The model under review builds one solid part; all positions refer to its coordinate system, in mm. A direction names the side the tool comes from. Give positions to 0.01 mm unless a question says otherwise; leave off trailing zeros. Loops run counter-clockwise (first coordinate to the right, second up) from the corner with the lowest first, then second, coordinate; pieces in that order, holes last. Notation, with made-up numbers: M 59.25,66.25 L 100.25,66.25 A18 ccw 100.25,92.25 Z; hole C 30,52.25 d5. An arc over 180 degrees is marked long. Return JSON: item names as keys, results as strings.
```python
from build123d import *

# Parameters (mm, degrees)
BOSS_EXTRUDE1_DEPTH      = 8
SKETCH2_R                = 1.5
CUT_EXTRUDE1_DEPTH       = 10
SKETCH3_R                = 1.5
CUT_EXTRUDE2_DEPTH       = 10
BOSS_EXTRUDE3_DEPTH      = 30
BOSS_EXTRUDE3_DEPTH_BACK = 8
SKETCH6_W                = 20
SKETCH6_H                = 10
FILLET3_R                = 12
SKETCH7_W                = 20
SKETCH7_H                = 30
BOSS_EXTRUDE4_DEPTH      = 2
CUT_EXTRUDE3_DEPTH       = 10
SKETCH9_R                = 5.5
CUT_EXTRUDE4_DEPTH       = 10
FILLET4_R                = 5
FILLET5_R                = 2


with BuildPart() as part:
    # Sketch1 → Boss-Extrude1 (new body)
    with BuildSketch(Plane.XY):
        with BuildLine():
            Line((-25, 10), (40, 10))
            ThreePointArc((40, 10), (50, 0), (40, -10))
            Line((40, -10), (-25, -10))
            Line((-25, -10), (-25, 10))
        make_face()
    extrude(amount=BOSS_EXTRUDE1_DEPTH)

    # Sketch2 → Cut-Extrude1 (cut)
    with BuildSketch(Plane.XY.offset(8)):
        with Locations((40, 0)):
            Circle(SKETCH2_R)
    extrude(amount=-CUT_EXTRUDE1_DEPTH, mode=Mode.SUBTRACT)

    # Sketch3 → Cut-Extrude2 (cut)
    with BuildSketch(Plane(origin=(0, 0, 0), x_dir=(-1, 0, 0), z_dir=(0, 0, -1))):
        with Locations((-15, 0)):
            Circle(SKETCH3_R)
    extrude(amount=-CUT_EXTRUDE2_DEPTH, mode=Mode.SUBTRACT)

    # Sketch6 → Boss-Extrude3 (add, two sides: drawn at the far end of the back side and taken through both)
    with BuildSketch(Plane(origin=(0, 0, 0), x_dir=(-1, 0, 0), z_dir=(0, 0, -1)).offset(-BOSS_EXTRUDE3_DEPTH_BACK)):
        with Locations((15, -15)):
            Rectangle(SKETCH6_W, SKETCH6_H)
    extrude(amount=BOSS_EXTRUDE3_DEPTH + BOSS_EXTRUDE3_DEPTH_BACK)

    # Fillet3
    # the kernel refuses this fillet: 12 mm, written as the material it adds along each edge
    with BuildSketch(Plane(origin=(-5, -10, 8), x_dir=(0, -1, 0), z_dir=(0, 0, -1))) as fillet3_piece_1:
        with BuildLine():
            CenterArc((12, -11.832159566), FILLET3_R, 99.594068227, 80.405931773)
            Line((0, -11.832159566), (0, 0))
            Line((0, 0), (10, 0))
        make_face()
    extrude(amount=8)

    # Sketch7 → Boss-Extrude4 (add)
    with BuildSketch(Plane(origin=(0, -10, 0), x_dir=(1, 0, 0), z_dir=(0, 1, 0))):
        with Locations((-15, 15)):
            Rectangle(SKETCH7_W, SKETCH7_H)
    extrude(amount=BOSS_EXTRUDE4_DEPTH)

    # Sketch8 → Cut-Extrude3 (cut)
    with BuildSketch(Plane.XZ.offset(20)):
        Polygon((-12.092828782, -7.012612723), (-20.463694682, -8.488622233), (-23.370865901, -16.47600951), (-17.907171218, -22.987387277), (-9.536305318, -21.511377767), (-6.629134099, -13.52399049), align=None)
    extrude(amount=-CUT_EXTRUDE3_DEPTH, mode=Mode.SUBTRACT)

    # Sketch9 → Cut-Extrude4 (cut)
    with BuildSketch(Plane.XZ.offset(10)):
        with Locations(Location((-15, -15, 0), (0, 0, 270))):
            Circle(SKETCH9_R)
    extrude(amount=-CUT_EXTRUDE4_DEPTH, mode=Mode.SUBTRACT)

    # Fillet4
    # the kernel refuses this fillet: 5 mm, written as the material it adds along each edge
    with BuildSketch(Plane(origin=(-5, -20, 0), x_dir=(1, 0, 0), z_dir=(0, 1, 0))) as fillet4_piece_1_section:
        with BuildLine():
            CenterArc((FILLET4_R, FILLET4_R), FILLET4_R, 180, 90)
            Line((0, FILLET4_R), (0, 0))
            Line((0, 0), (FILLET4_R, 0))
        make_face()
    fillet4_piece_1 = extrude(amount=12, mode=Mode.PRIVATE)
    fillet4_piece_1 = fillet4_piece_1 - Plane(origin=(6.832159566, -22, 0), x_dir=(0, -1, 0), z_dir=(0, 0, 1)) * Cylinder(12, 44, mode=Mode.PRIVATE)
    add(fillet4_piece_1)
    with BuildSketch(Plane(origin=(-25, -8, 0), x_dir=(0, 1, 0), z_dir=(1, 0, 0))) as fillet4_piece_2:
        with BuildLine():
            CenterArc((FILLET4_R, -FILLET4_R), FILLET4_R, 90, 90)
            Line((0, -FILLET4_R), (0, 0))
            Line((0, 0), (FILLET4_R, 0))
        make_face()
    extrude(amount=20)
    with BuildSketch(Plane(origin=(-5, -20, 0), x_dir=(1, 0, 0), z_dir=(0, 1, 0))) as fillet4_piece_3a_section:
        with BuildLine():
            CenterArc((FILLET4_R, FILLET4_R), FILLET4_R, 180, 90)
            Line((0, FILLET4_R), (0, 0))
            Line((0, 0), (FILLET4_R, 0))
        make_face()
    fillet4_piece_3a = extrude(amount=24.5, mode=Mode.PRIVATE)
    fillet4_piece_3a = split(fillet4_piece_3a, bisect_by=Plane(origin=(-5, -8, 0), z_dir=(0, 1, 0)), keep=Keep.TOP, mode=Mode.PRIVATE)
    with BuildSketch(Plane(origin=(-25, -8, 0), x_dir=(0, 1, 0), z_dir=(1, 0, 0))) as fillet4_piece_3b_section:
        with BuildLine():
            CenterArc((FILLET4_R, -FILLET4_R), FILLET4_R, 90, 90)
            Line((0, -FILLET4_R), (0, 0))
            Line((0, 0), (FILLET4_R, 0))
        make_face()
    fillet4_piece_3b = extrude(amount=32.5, mode=Mode.PRIVATE)
    fillet4_piece_3b = split(fillet4_piece_3b, bisect_by=Plane(origin=(-5, -8, 0), z_dir=(1, 0, 0)), keep=Keep.TOP, mode=Mode.PRIVATE)
    fillet4_piece_3 = fillet4_piece_3a & fillet4_piece_3b
    add(fillet4_piece_3)

    # Fillet5
    fillet5_edges = [part.edges().sort_by_distance(p)[0] for p in [
        (-15, -20, 8),
        (-25, -14, -30),
        (-5, -14, -30),
        (-25, 10, 4),
    ]]
    fillet(fillet5_edges, radius=FILLET5_R)


solid = part.part
```
1) Consider section B-B on z = -15. Write out the cut boundary in (x, y).
From the geometry:
{"outline": "M -25,-20 L -22.83,-20 L -22.83,-10 L -20.5,-10 L -20.5,-8 L -25,-8 Z; M -9.5,-10 L -7.17,-10 L -7.17,-20 L -5,-20 L -5,-8 L -9.5,-8 Z"}
2) Wall thickness on L1, parallel to Y at x = 15, z = 2; L2, parallel to X at y = -8.9, z = -15; L3, parallel to Y at x = 8, z = 3.5: over which ranges is each line inside the solid? List them lowest first. Write a range as from..to.
From the geometry:
{"L1": "-10..-1.5, 1.5..10", "L2": "-25..-20.5, -9.5..-5", "L3": "-10..10"}
3) The part is to be moulded in two halves that separate along Z. For faces 4 (the face through (-24.43, -14.08, -29.4)), 5 (the face through (-8.1, -15.07, -17.57)), 6 (the face through (-25, -12, -6)), say which applies: released by +Z, released by -Z, zero draft, split by the parting line, or undercut.
From the geometry:
{"face 4": "released by -Z", "face 5": "undercut", "face 6": "zero draft"}
4) Insertion check: pin 1 (1.5 mm diameter, centred on x = 32, y = -0.5, fed in from -Z); pin 2 (4 mm diameter, centred on x = 30, z = 3, fed in from -Y); pin 3 (3.5 mm diameter, centred on y = -14.5, z = -13.5, fed in from +X). Each pin has a flat end and moves straight along its axis. Give the tip position at first contact, or say it passes through.
From the geometry:
{"pin 1": "z = 0", "pin 2": "y = -10", "pin 3": "x = -5"}
5) Tool access review of faces 1 (the face through (8, 10, 4)), 2 (the face through (-13.78, -15.07, -22.26)), 3 (the face through (-17.1, -8, -20.5)): name each direction out of +Z, -Z, +X, -X, +Y, -Y from which nothing blocks a thin tool from reaching the whole face with its end or side.
From the geometry:
{"face 1": "+Z, -Z, +X, -X, +Y", "face 2": "-Y", "face 3": "-Z, +X, -X, +Y"}
6) Consider section D-D on x = -13. Write out the cut boundary in (y, z), then the cut area to 3 significant figures.
From the geometry:
{"outline": "M -20,-30 L -8,-30 L -8,-20.12 L -10,-20.12 L -10,-22.12 L -20,-22.12 Z; M -20,-7.17 L -10,-7.17 L -10,-9.88 L -8,-9.88 L -8,-5 A5 cw -3,0 L 10,0 L 10,8 L -18,8 A2 ccw -20,6 Z", "area": "435 mm²"}
7) Consider section C-C on y = -17. Write out the cut boundary in (x, z), then the cut area to 3 significant figures.
From the geometry:
{"outline": "M -25,-28 A2 ccw -23,-30 L -7,-30 A2 ccw -5,-28 L -5,-5 A5 cw -4.08,-2.1 L -4.08,8 L -25,8 Z; hole M -23.37,-16.48 L -17.91,-22.99 L -9.54,-21.51 L -6.63,-13.52 L -12.09,-7.01 L -20.46,-8.49 Z", "area": "581 mm²"}
8) Consider section A-A on x = 15. Write out the cut boundary in (y, z).
From the geometry:
{"outline": "M -10,0 L -1.5,0 L -1.5,8 L -10,8 Z; M 1.5,0 L 10,0 L 10,8 L 1.5,8 Z"}
